from build123d import *

# Parameters (mm, degrees)
ESQUISSE1_W      = 42.2
ESQUISSE1_H      = 42.2
EXTRUSION1_DEPTH = 41.1
ESQUISSE2_R      = 11
EXTRUSION2_DEPTH = 2
ESQUISSE3_R      = 2.5
EXTRUSION3_DEPTH = 18
ESQUISSE4_R      = 1.5
EXTRUSION4_DEPTH = 4


with BuildPart() as part:
    # Esquisse1 → Extrusion1 (new body)
    with BuildSketch(Plane.XY):
        with Locations((7.023594794, 4.422730203)):
            Rectangle(ESQUISSE1_W, ESQUISSE1_H)
    extrude(amount=EXTRUSION1_DEPTH)

    # Esquisse2 → Extrusion2 (add)
    with BuildSketch(Plane.XY.offset(41.1)):
        with Locations(Location((7.023594794, 4.422730203, 0), (0, 0, 180))):
            Circle(ESQUISSE2_R)
    extrude(amount=EXTRUSION2_DEPTH)

    # Esquisse3 → Extrusion3 (add)
    with BuildSketch(Plane.XY.offset(43.1)):
        with Locations((7.023594794, 4.422730203)):
            Circle(ESQUISSE3_R)
    extrude(amount=EXTRUSION3_DEPTH)

    # Esquisse4 → Extrusion4 (cut)
    with BuildSketch(Plane.XY.offset(41.1)):
        with Locations((-8.476405206, 19.922730203)):
            Circle(ESQUISSE4_R)
        with Locations(Location((22.523594794, 19.922730203, 0), (0, 0, 180))):
            Circle(ESQUISSE4_R)
        with Locations((22.523594794, -11.077269797)):
            Circle(ESQUISSE4_R)
        with Locations(Location((-8.476405206, -11.077269797, 0), (0, 0, 180))):
            Circle(ESQUISSE4_R)
    extrude(amount=-EXTRUSION4_DEPTH, mode=Mode.SUBTRACT)


solid = part.part
Geometry check sheet. Reference: the model listing, model coordinates, mm. A direction names the side the tool comes from. Give positions to 0.01 mm unless a question says otherwise; leave off trailing zeros. Order: outer loops, then holes, each group sorted by start corner. A loop starts at its lowest first (then second) coordinate and runs counter-clockwise, first axis right, second up.
1) Tool access check on faces 1 (the flat face through (7, -16.677, 20)), 2 (the cylindrical face through (21.025, -11.011, 39.128)). Record the directions out of +Z, -Z, +X, -X, +Y, -Y that give a thin tool (end or side, any length) a straight path to the whole face; none if there is none.
Results are:
face 1: +Z, -Z, +X, -X, -Y
face 2: +Z
2) Gauge pin test, flat ends, axial feed: pin 1 (1.5 mm diameter, centred on x = 9, z = 45, fed in from +Y); pin 2 (0.9 mm diameter, centred on x = -9, y = 19.5, fed in from +Z); pin 3 (3.5 mm diameter, centred on x = -8.5, y = -11, fed in from +Z). Record the tip position at first contact, or that the pin passes through.
Results are:
pin 1: stops at y = 6.6
pin 2: stops at z = 37.1
pin 3: stops at z = 41.1
3) Draft check along X on faces 3 (the flat face through (28.124, 4, 20)), 4 (the flat face through (-8, 20, 37.1)), 5 (the flat face through (-14.076, 4, 20)). Enter one of: released by +X, released by -X, zero draft, split by the parting line, or undercut.
Results are:
face 3: released by +X
face 4: undercut
face 5: released by -X
4) Cross-section at D-D (z = 54.5). Record the boundary of the cut face in (x, y).
Results are:
outline: circle Ø5 at (7.02, 4.42)
5) Material ranges on probe 1 along Z at (x, y) = (26, -13.5); probe 2 along Z at (x, y) = (22.5, -11); probe 3 along X at (y, z) = (5, 53), recorded low to high.
Results are:
probe 1: z = 0 to 41.1
probe 2: z = 0 to 37.1
probe 3: x = 4.59 to 9.46
6) Cross-section at A-A (z = 38.5). Record the boundary of the cut face in (x, y), then the cut area to 3 significant figures.
Results are:
outline: (-14.08, -16.68) - (28.12, -16.68) - (28.12, 25.52) - (-14.08, 25.52) - close; hole circle Ø3 at (-8.48, -11.08); hole circle Ø3 at (-8.48, 19.92); hole circle Ø3 at (22.52, -11.08); hole circle Ø3 at (22.52, 19.92)
area: 1,750 mm2
7) Cross-section at C-C (y = 14.5). Record the boundary of the cut face in (x, z), then the cut area to 3 significant figures.
Results are:
outline: (-14.08, 0) - (28.12, 0) - (28.12, 41.1) - (11.43, 41.1) - (11.43, 43.1) - (2.61, 43.1) - (2.61, 41.1) - (-14.08, 41.1) - close
area: 1,750 mm2
8) Cross-section at B-B (x = 17). Record the boundary of the cut face in (y, z).
Results are:
outline: (-16.68, 0) - (25.52, 0) - (25.52, 41.1) - (9.06, 41.1) - (9.06, 43.1) - (-0.21, 43.1) - (-0.21, 41.1) - (-16.68, 41.1) - close
